from build123d import *

# Parameters (mm, degrees)
SKETCH1_W                                    = 320
SKETCH1_H                                    = 220
BOSS_EXTRUDE1_DEPTH                          = 15
FILLET2_R                                    = 1
CBORE_FOR_M5_HEX_SOCKET_HEAD_CAP_SCR_2_COUNT = 2
CBORE_FOR_M5_HEX_SOCKET_HEAD_CAP_SCR_2_PITCH = 200
CBORE_FOR_M5_HEX_SOCKET_HEAD_CAP_SCR_3_COUNT = 2
CBORE_FOR_M5_HEX_SOCKET_HEAD_CAP_SCR_3_PITCH = 344.093010682
CBORE_FOR_M5_HEX_SOCKET_HEAD_CAP_SCR_4_COUNT = 2
CBORE_FOR_M5_HEX_SOCKET_HEAD_CAP_SCR_4_PITCH = 280
SKETCH7_W                                    = 10
SKETCH7_H                                    = 11.203973801
CUT_EXTRUDE1_DEPTH                           = 321


with BuildPart() as part:
    # Sketch1 → Boss-Extrude1 (new body)
    with BuildSketch(Plane(origin=(0, 0, 0), x_dir=(1, 0, 0), z_dir=(0, 1, 0))):
        Rectangle(SKETCH1_W, SKETCH1_H)
    extrude(amount=BOSS_EXTRUDE1_DEPTH)

    # Fillet2
    fillet2_edges = [part.edges().sort_by_distance(p)[0] for p in [
        (-160, 7.5, -110),
        (160, 7.5, -110),
        (160, 7.5, 110),
        (-160, 7.5, 110),
    ]]
    fillet(fillet2_edges, radius=FILLET2_R)

    # Sketch5 → CBORE for M5 Hex Socket Head Cap Screw2 (revolve, cut)
    with BuildSketch(Plane(origin=(-140, 15, -100), x_dir=(0, 0, 1), z_dir=(1, 0, 0))):
        Polygon((0, 0), (0, 15), (2.75, 15), (2.75, 6), (4.25, 6), (4.25, 0.775), (5.025, 0), align=None)
    cbore_for_m5_hex_socket_head_cap_screw2 = revolve(axis=Axis((-140, 21.35, -100), (0, -1, 0)), mode=Mode.SUBTRACT)

    # CBORE for M5 Hex Socket Head Cap Scr 2: CBORE for M5 Hex Socket Head Cap Screw2 ×2
    with Locations(*[(0, 0, i * CBORE_FOR_M5_HEX_SOCKET_HEAD_CAP_SCR_2_PITCH) for i in range(1, CBORE_FOR_M5_HEX_SOCKET_HEAD_CAP_SCR_2_COUNT)]):
        add(cbore_for_m5_hex_socket_head_cap_screw2, mode=Mode.SUBTRACT)

    # CBORE for M5 Hex Socket Head Cap Scr 3: CBORE for M5 Hex Socket Head Cap Screw2 ×2
    with Locations(*[Vector(0.813733471, 0, 0.581238194) * (i * CBORE_FOR_M5_HEX_SOCKET_HEAD_CAP_SCR_3_PITCH) for i in range(1, CBORE_FOR_M5_HEX_SOCKET_HEAD_CAP_SCR_3_COUNT)]):
        add(cbore_for_m5_hex_socket_head_cap_screw2, mode=Mode.SUBTRACT)

    # CBORE for M5 Hex Socket Head Cap Scr 4: CBORE for M5 Hex Socket Head Cap Screw2 ×2
    with Locations(*[(i * CBORE_FOR_M5_HEX_SOCKET_HEAD_CAP_SCR_4_PITCH, 0, 0) for i in range(1, CBORE_FOR_M5_HEX_SOCKET_HEAD_CAP_SCR_4_COUNT)]):
        add(cbore_for_m5_hex_socket_head_cap_screw2, mode=Mode.SUBTRACT)

    # Sketch7 → Cut-Extrude1 (cut, through all)
    with BuildSketch(Plane.ZY.offset(160)):
        with Locations((-88, 9.3980131)):
            Rectangle(SKETCH7_W, SKETCH7_H)
        with Locations((8, 9.3980131)):
            Rectangle(SKETCH7_W, SKETCH7_H)
        with Locations((-68, 9.3980131)):
            Rectangle(SKETCH7_W, SKETCH7_H)
        with Locations((-48, 9.3980131)):
            Rectangle(SKETCH7_W, SKETCH7_H)
        with Locations((-28, 9.3980131)):
            Rectangle(SKETCH7_W, SKETCH7_H)
        with Locations((-8, 9.3980131)):
            Rectangle(SKETCH7_W, SKETCH7_H)
        with Locations((28, 9.3980131)):
            Rectangle(SKETCH7_W, SKETCH7_H)
        with Locations((48, 9.3980131)):
            Rectangle(SKETCH7_W, SKETCH7_H)
        with Locations((68, 9.3980131)):
            Rectangle(SKETCH7_W, SKETCH7_H)
        with Locations((88, 9.3980131)):
            Rectangle(SKETCH7_W, SKETCH7_H)
    extrude(amount=-CUT_EXTRUDE1_DEPTH, mode=Mode.SUBTRACT)


solid = part.part
CAD build for the part. Positions are in the model's coordinates, mm. A direction names the side the tool comes from. Round coordinates to 2 decimals unless told otherwise and drop trailing zeros. Loops run counter-clockwise (first coordinate to the right, second up) from the corner with the lowest first, then second, coordinate; pieces in that order, holes last.
(1) Drop flat-ended pins along their axis: pin 1 (4.5 mm diameter, centred on x = -140, z = 100, fed in from -Y); pin 2 (5 mm diameter, centred on x = 33, z = -69, fed in from +Y); pin 3 (2.5 mm diameter, centred on x = -141.5, z = -101, fed in from +Y). Give the stop position or say it passes through.
(2) Which spindle directions (+Z, -Z, +X, -X, +Y, -Y) get a long thin tool onto all of the face, cutting with end or side? Do faces 3 (the flat face through (140, 9, 97)), 4 (the flat face through (-2, 15, 18)), 5 (the flat face through (-2, 9, 83)). Say none if no direction does.
(3) Wall check: line 1 along Z through (x, y) = (140, 3.25); line 2 along X through (y, z) = (13, -100); line 3 along X through (y, z) = (3.25, -100). Give the ranges that are in metal, low to high.
(4) Cut at A-A (z = -87). Give the cut face in (x, y), plus the area to 3 significant figures.
(5) Two-plate mould, pull along Z, no slides. Class faces 1 (the flat face through (-2, 15, -102)), 2 (the flat face through (-2, 3.796, 48)): +Z half, -Z half, draft (parallel to the pull), parting line (faces both ways), or undercut.
Findings below:
1. pin 1: passes through
1. pin 2: stops at y = 3.8
1. pin 3: stops at y = 9
2. face 3: +Y
2. face 4: +Z, -Z, +X, -X, +Y
2. face 5: +X, -X, +Y
3. line 1: z = -110 to -102.75, -97.25 to 97.25, 102.75 to 110
3. line 2: x = -160 to -144.25, -135.75 to 135.75, 144.25 to 160
3. line 3: x = -160 to -142.75, -137.25 to 137.25, 142.75 to 160
4. outline: (-160, 0) - (160, 0) - (160, 3.8) - (-160, 3.8) - close
4. area: 1,210 mm2
5. face 1: draft
5. face 2: undercut
